Source: CAD feature listing. Evaluate the final solid. Frame: model axes, mm. A direction names the side the tool comes from. Round coordinates to 2 decimals unless told otherwise and drop trailing zeros. Write each loop counter-clockwise with the first axis right and the second up, starting at its lowest first coordinate (ties: lowest second). Pieces come first, ordered by that corner, then holes. Notation, with made-up numbers: M 20.25,50.5 L 71.25,50.5 A28 ccw 71.25,75.5 Z; hole C 60,73 d10. An arc over 180 degrees is marked long. Answer in a Markdown table with one row per item.
Autodesk Inventor part; units mm, degrees
ref_plane "bolt_XY" through (0, 0, 0) normal (1, 0, 0) x (0, 0, -1)
ref_plane "bolt_YZ" through (0, 0, 0) normal (0, 0, -1) x (0, 1, 0)
ref_plane "bolt_ZX" through (0, 0, 0) normal (0, 1, 0) x (1, 0, 0)
sketch "Sketch_2" plane through (0, 0, 0) normal (0, 0, 1) x (1, 0, 0)
  line L0 (45, 0) -> (-5, 0)
  line L1 (-5, 0) -> (-5, 3.6833)
  line L2 (-5, 3.6833) -> (-4.4333, 4.25)
  line L3 (-4.4333, 4.25) -> (0, 4.25)
  line L4 (0, 4.25) -> (0, 2.5)
  line L5 (0, 2.5) -> (44.5095, 2.5)
  line L6 (44.5095, 2.5) -> (45, 2.0095)
  line L7 (45, 2.0095) -> (45, 0)
  line L8 (45, 0) -> (-5, 0)
revolve "Revolution1" add sketch "Sketch_2" angle 360 about axis through (45, 0, 0) along (1, 0, 0)
thread "Thread1"
sketch "Sketch2" plane through (-5, 0, 0) normal (-1, 0, 0) x (0, 0, 1)
  point P0 (0, 0)
hole "Hole1" at (-5, 0, 0) direction (1, 0, 0) diameter 4 depth 2.5 tip angle 150
sketch "Sketch_3" plane through (-5, 0, 0) normal (1, 0, 0) x (0, 0, -1)
  line L0 (-2, -1.1547) -> (0, -2.3094)
  line L1 (0, -2.3094) -> (2, -1.1547)
  line L2 (2, -1.1547) -> (2, 1.1547)
  line L3 (2, 1.1547) -> (0, 2.3094)
  line L4 (0, 2.3094) -> (-2, 1.1547)
  line L5 (-2, 1.1547) -> (-2, -1.1547)
extrude "Extrusion1" cut sketch "Sketch_3" along normal blind 2.5
ref_plane "bolt_XY" through (0, 0, 0) normal (1, 0, 0) x (0, 0, -1)
ref_plane "bolt_YZ" through (0, 0, 0) normal (0, 0, -1) x (0, 1, 0)
ref_plane "bolt_ZX" through (0, 0, 0) normal (0, 1, 0) x (1, 0, 0)
ref_plane "nut_XY" through (45, 0, 0) normal (1, 0, 0) x (0, 0, -1)
ref_plane "nut_YZ" through (45, 0, 0) normal (0, 0, -1) x (0, 1, 0)
ref_plane "nut_ZX" through (45, 0, 0) normal (0, 1, 0) x (1, 0, 0)
properties part number "SCB5-45"
Q1. Material intervals for probe 1 along Y at (x, z) = (15, -1.5); probe 2 along X at (y, z) = (2.25, 1.5); probe 3 along X at (y, z) = (2, 3.5), sorted ascending.
Solutions:
| item | result |
|---|---|
| probe 1 | y = -2 to 2 |
| probe 2 | x = -5 to 0 |
| probe 3 | x = -4.65 to 0 |
Q2. Access query for faces 1 (the cylindrical face through (-2.186, 2.285, 3.584)), 2 (the flat face through (0, 2, -2)), 3 (the flat face through (-3.768, 1.724, -1.014)). Directions: +Z, -Z, +X, -X, +Y, -Y. A direction counts if a zero-diameter tool reaches every point of the face in a straight line with its end or side. Return the directions, or none.
Solutions:
| item | result |
|---|---|
| face 1 | +X, -X |
| face 2 | +X |
| face 3 | -X |
Q3. Pull-direction query (Z, two-part tool) for faces 4 (the cylindrical face through (22.57, -0.54, -2.44)), 5 (the flat face through (-5, 2, -2)), 6 (the flat face through (-4, 0, 2)); classes: pulls with the +Z half, pulls with the -Z half, needs draft (parallel to the pull), parting line crosses it, or undercut.
Solutions:
| item | result |
|---|---|
| face 4 | parting line crosses it |
| face 5 | needs draft |
| face 6 | undercut |
Q4. Contact query for flat-ended pins moving along their axis: pin 1 Ø1.5 at (x, z) = (31, 0) entering from -Y; pin 2 Ø0.5 at (y, z) = (-1, -1.5) entering from -X; pin 3 Ø5 at (x, y) = (36.5, 2.5) entering from +Z. Output: stop coordinate, or through.
Solutions:
| item | result |
|---|---|
| pin 1 | stops at y = -2.5 |
| pin 2 | stops at x = -2.5 |
| pin 3 | stops at z = 2.5 |
Q5. Section A-A (x = 0.5). Return loops of the section in (y, z), and give its area (3 significant figures).
Solutions:
| item | result |
|---|---|
| outline | C 0,0 d5 |
| area | 19.6 mm2 |
